```python
from build123d import *

# Parameters (mm, degrees)
F1_R = 1


with BuildPart() as f2:
    # F2: sweep along a path in F0
    with BuildLine(Plane.XZ) as f2_path:
        Line((0, 0), (-35, 0))
        ThreePointArc((-35, 0), (-45.606602, -4.393398), (-50, -15))
        Line((-50, -15), (-50, -145))
    # F1 (on Right) → F2 (sweep)
    with BuildSketch(Plane.YZ):
        with Locations((0, 1)):
            Circle(F1_R)
    sweep(path=f2_path.line)

    # F3: F2 across plane


with BuildPart() as f2_1:
    add(f2.part)
    add(f2.part.mirror(Plane.YZ))


solid = f2_1.part
```
Verification items for the finished model (mm, model axes). Give positions to 0.01 mm unless a question says otherwise; leave off trailing zeros. Write each loop counter-clockwise with the first axis right and the second up, starting at its lowest first coordinate (ties: lowest second). Pieces come first, ordered by that corner, then holes. Notation, with made-up numbers: (16, 61) - (25, 61) arc R14 cw to (25, 76) - close; hole circle Ø11 at (-40, -37). An arc over 180 degrees is marked (long way). Put each result on its own line as item: value.
Q1. Depth check by flat-ended pin: P1, Ø1, axis at x = -41.5, y = -0.5, coming from the +Z side; P2, Ø1, axis at x = 40.5, y = 0.5, coming from the -Z side. Enter the tip coordinate at first touch or a pass-through.
Result:
P1: z = 0.85
P2: z = -1.19
Q2. Scan lines: probe 1 along X at (y, z) = (-0.25, -79.5); probe 2 along X at (y, z) = (0.4, -9.5); probe 3 along Z at (x, y) = (-31, 0.15). Record each from-to range of solid material in increasing order. Write a range as from..to.
Result:
probe 1: -51.97..-50.03, 50.03..51.97
probe 2: -51..-49.04, 49.04..51
probe 3: 0.01..1.99
Q3. Section check A-A on x = 24. Record the cut outline in (y, z).
Result:
outline: circle Ø2 at (0, 1)
